Design review of the part built by this model. Coordinates are the model's own, in mm. Face numbers are marked on the shaded views. A direction names the side the tool comes from. Coordinates: 2 decimals unless noted, no trailing zeros. Write each loop counter-clockwise with the first axis right and the second up, starting at its lowest first coordinate (ties: lowest second). Pieces come first, ordered by that corner, then holes.
Q1. Add section A-A, the plane x = -32.03. Give the boundary of the cut face in (y, z) (3 decimals).
Q2. Add section B-B, the plane x = -51. Give the boundary of the cut face in (y, z) (3 decimals), plus the area to 3 significant figures.
Q3. The part is to be moulded in two halves that separate along X. For the marked faces 1, 2 and 3, say which applies: +X half, -X half, draft (parallel to the pull), parting line (faces both ways), or undercut.
Q4. Clearance check with a flat-ended pin moving along its axis: pin 1 Ø4 at (x, y) = (-49, 6) entering from -Z. State where the tip first meets the part, or that it passes through.
Q5. Add section C-C, the plane z = -12. Give the number of separate pieces and of enclosed holes in the cut face, plus the area to 3 significant figures.
Q6. To check wall thickness, follow probe 1 along Z at (x, y) = (-47, 10.5); probe 2 along Y at (x, z) = (-2.5, -6.75) (3 decimals); probe 3 along Y at (x, z) = (-32.03, -0.5) (3 decimals). State the ranges of each line that lie inside material, in increasing order.
Q7. Machinability: for the marked faces 4 and 5, which of the approach directions +Z, -Z, +X, -X, +Y, -Y give a long, thin tool a straight path to every point of the face, cutting with its end or side? Answer none if there is none.
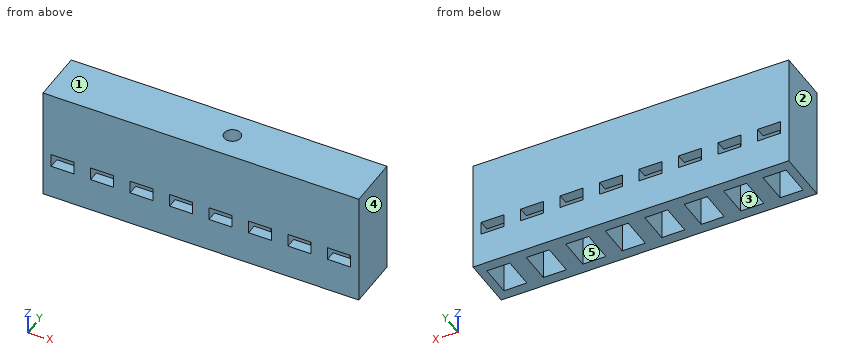
from build123d import *

# Parameters (mm, degrees)
SKETCH1_W           = 72
SKETCH1_H           = 22
BOSS_EXTRUDE1_DEPTH = 12
SKETCH2_W           = 5.25
SKETCH2_H           = 3
CUT_EXTRUDE1_DEPTH  = 77.23647421
LPATTERN2_COUNT     = 8
LPATTERN2_PITCH     = 9
SKETCH3_W           = 5.25
SKETCH3_H           = 7.25
CUT_EXTRUDE2_DEPTH  = 77.23647421
LPATTERN3_COUNT     = 8
LPATTERN3_PITCH     = 9
SKETCH4_W           = 72
SKETCH4_H           = 12
BOSS_EXTRUDE2_DEPTH = 4
SKETCH11_W          = 72
SKETCH11_H          = 12
BOSS_EXTRUDE3_DEPTH = 4
SKETCH12_R          = 1.865
CUT_EXTRUDE9_DEPTH  = 6


with BuildPart() as part:
    # Sketch1 → Boss-Extrude1 (new body)
    with BuildSketch(Plane(origin=(0, 0, 0), x_dir=(1, 0, 0), z_dir=(0, 1, 0))):
        with Locations((-36, 11)):
            Rectangle(SKETCH1_W, SKETCH1_H)
    extrude(amount=BOSS_EXTRUDE1_DEPTH)

    # Sketch2 → Cut-Extrude1 (cut, through all)
    with BuildSketch(Plane(origin=(0, 12, 0), x_dir=(1, 0, 0), z_dir=(0, 1, 0))):
        with Locations((-67.5, 12.7)):
            Rectangle(SKETCH2_W, SKETCH2_H)
    cut_extrude1 = extrude(amount=-CUT_EXTRUDE1_DEPTH, mode=Mode.SUBTRACT)

    # LPattern2: Cut-Extrude1 ×8
    with Locations(*[(i * LPATTERN2_PITCH, 0, 0) for i in range(1, LPATTERN2_COUNT)]):
        add(cut_extrude1, mode=Mode.SUBTRACT)

    # Sketch3 → Cut-Extrude2 (cut, through all)
    with BuildSketch(Plane(origin=(0, 0, -22), x_dir=(-1, 0, 0), z_dir=(0, 0, -1))):
        with Locations((67.5, 6)):
            Rectangle(SKETCH3_W, SKETCH3_H)
    cut_extrude2 = extrude(amount=-CUT_EXTRUDE2_DEPTH, mode=Mode.SUBTRACT)

    # LPattern3: Cut-Extrude2 ×8
    with Locations(*[(i * LPATTERN3_PITCH, 0, 0) for i in range(1, LPATTERN3_COUNT)]):
        add(cut_extrude2, mode=Mode.SUBTRACT)

    # Sketch4 → Boss-Extrude2 (add)
    with BuildSketch(Plane.XY):
        with Locations((-36, 6)):
            Rectangle(SKETCH4_W, SKETCH4_H)
    extrude(amount=-BOSS_EXTRUDE2_DEPTH)

    # Sketch11 → Boss-Extrude3 (add)
    with BuildSketch(Plane.XY):
        with Locations((-36, 6)):
            Rectangle(SKETCH11_W, SKETCH11_H)
    extrude(amount=BOSS_EXTRUDE3_DEPTH)

    # Sketch12 → Cut-Extrude9 (cut)
    with BuildSketch(Plane.XY.offset(4)):
        with Locations((-32.03, 6)):
            Circle(SKETCH12_R)
    extrude(amount=-CUT_EXTRUDE9_DEPTH, mode=Mode.SUBTRACT)


solid = part.part
Here are the results:
1. outline: (0, -22) - (2.375, -22) - (2.375, -14.2) - (0, -14.2) - close; (0, -11.2) - (2.375, -11.2) - (2.375, -4) - (9.625, -4) - (9.625, -11.2) - (12, -11.2) - (12, 4) - (7.865, 4) - (7.865, -2) - (4.135, -2) - (4.135, 4) - (0, 4) - close; (9.625, -22) - (12, -22) - (12, -14.2) - (9.625, -14.2) - close
2. outline: (0, -22) - (2.375, -22) - (2.375, -14.2) - (0, -14.2) - close; (0, -11.2) - (2.375, -11.2) - (2.375, -4) - (9.625, -4) - (9.625, -11.2) - (12, -11.2) - (12, 4) - (0, 4) - close; (9.625, -22) - (12, -22) - (12, -14.2) - (9.625, -14.2) - close
2. area: 167 mm2
3. face 1: draft
3. face 2: -X half
3. face 3: undercut
4. pin 1: stops at z = -4
5. separate pieces: 9
5. enclosed holes: 0
5. area: 360 mm2
6. probe 1: z = -22 to -14.2, -11.2 to 4
6. probe 2: y = 0 to 2.375, 9.625 to 12
6. probe 3: y = 0 to 4.135, 7.865 to 12
7. face 4: +Z, -Z, +X, +Y, -Y
7. face 5: -Z
